from build123d import *

# Parameters (mm, degrees)
SKETCH_3_R               = 5
SKETCH_4_R               = 2
CUT_EXTRUDE_1_DEPTH      = 10
CUT_EXTRUDE_1_DEPTH_BACK = 10
SKETCH_6_R               = 2
CUT_EXTRUDE_3_DEPTH      = 129


with BuildPart() as part:
    # Sweep 1: sweep along a path in Sketch 1
    with BuildLine(Plane.XY) as sweep_1_path:
        Line((0, 0), (-40, 0))
        ThreePointArc((-40, 0), (-47.071067812, 2.928932188), (-50, 10))
        Line((-50, 10), (-50, 90))
        ThreePointArc((-50, 90), (-47.071067812, 97.071067812), (-40, 100))
        Line((-40, 100), (100, 100))
    # Sketch 3 → Sweep 1 (sweep)
    with BuildSketch(Plane(origin=(0, 0, 0), x_dir=(0, 0, -1), z_dir=(1, 0, 0))):
        Circle(SKETCH_3_R)
    sweep(path=sweep_1_path.line)

    # Sketch 4 → Cut-Extrude 1 (cut, two sides)
    with BuildSketch(Plane.XY) as cut_extrude_1_sk:
        with Locations((-10, 0)):
            Circle(SKETCH_4_R)
    extrude(amount=CUT_EXTRUDE_1_DEPTH, mode=Mode.SUBTRACT)
    extrude(cut_extrude_1_sk.sketch, amount=-CUT_EXTRUDE_1_DEPTH_BACK, mode=Mode.SUBTRACT)

    # Sketch 6 → Cut-Extrude 3 (cut)
    with BuildSketch(Plane(origin=(0, 70, 0), x_dir=(1, 0, 0), z_dir=(0, 1, 0))):
        with Locations((70, 0)):
            Circle(SKETCH_6_R)
        with Locations((-10, 0)):
            Circle(SKETCH_6_R)
    extrude(amount=CUT_EXTRUDE_3_DEPTH, mode=Mode.SUBTRACT)


solid = part.part
CAD build for the part. Positions are in the model's coordinates, mm. A direction names the side the tool comes from. Round coordinates to 2 decimals unless told otherwise and drop trailing zeros. Write each loop counter-clockwise with the first axis right and the second up, starting at its lowest first coordinate (ties: lowest second). Pieces come first, ordered by that corner, then holes.
(1) Slice it at D-D, the plane x = 89.5. Write the cut outline in (y, z), and give its area (3 significant figures).
(2) Probe line 1 along Y through (x, z) = (-10, 0); line 2 along X through (y, z) = (98.5, 0); line 3 along Y through (x, z) = (-10, -2.5). List the from-to ranges inside material, lowest first.
(3) Drop flat-ended pins along their axis: P1, Ø12, axis at x = 4.5, y = 13.5, coming from the -Z side; P2, Ø1, axis at y = 48.5, z = 2.5, coming from the +X side; P3, Ø4, axis at x = -10.5, z = 4, coming from the -Y side; P4, Ø3, axis at y = -2, z = -2, coming from the +X side. Give the stop position or say it passes through.
(4) Slice it at B-B, the plane x = -23.5. Write the cut outline in (y, z), and give its area (3 significant figures).
(5) Slice it at A-A, the plane z = 0. Write the cut outline in (x, y), and give its area (3 significant figures).
(6) Slice it at C-C, the plane y = 82. Write the cut outline in (x, z), and give its area (3 significant figures).
(7) 3-axis set-ups, long thin cutter, end or side, ignore diameter. For faces 5 (the face through (0, 0, 0)), 6 (the face through (100, 100, 0)), 7 (the face through (-20.28, 1.915, -4.619)), 8 (the face through (-54.957, 50.56, 0.651)): which of +Z, -Z, +X, -X, +Y, -Y reach the whole face in a straight line?
(8) Mould opens along Z. For faces 1 (the face through (71.908, 99.93, -0.601)), 2 (the face through (-11.6, -1.2, 0.1)), 3 (the face through (-11.6, 99.9, 1.2)), 4 (the face through (30.98, 95.12, 1.08)) say: pulls with the +Z half, pulls with the -Z half, needs draft (parallel to the pull), parting line crosses it, or undercut.
From the geometry:
1. outline: circle Ø10 at (100, 0)
1. area: 78.5 mm2
2. line 1: y = -5 to -2, 2 to 5
2. line 2: x = -52.36 to -12, -8 to 68, 72 to 100
2. line 3: y = -4.33 to -2, 2 to 4.33, 95.67 to 104.33
3. P1: passes through
3. P2: stops at x = -45.42
3. P3: stops at y = -4.58
3. P4: stops at x = 0
4. outline: circle Ø10 at (0, 0); circle Ø10 at (100, 0)
4. area: 157 mm2
5. outline: (-55, 10) arc R15 ccw to (-40, -5) - (0, -5) - (0, 5) - (-40, 5) arc R5 cw to (-45, 10) - (-45, 90) arc R5 cw to (-40, 95) - (-12, 95) - (-12, 105) - (-40, 105) arc R15 ccw to (-55, 90) - close; (-8, 95) - (68, 95) - (68, 105) - (-8, 105) - close; (72, 95) - (100, 95) - (100, 105) - (72, 105) - close; hole circle Ø4 at (-10, 0)
5. area: 2,820 mm2
6. outline: circle Ø10 at (-50, 0)
6. area: 78.5 mm2
7. face 5: +Z, -Z, +X, -Y
7. face 6: +Z, -Z, +X, +Y, -Y
7. face 7: +X
7. face 8: none
8. face 1: undercut
8. face 2: needs draft
8. face 3: undercut
8. face 4: parting line crosses it
